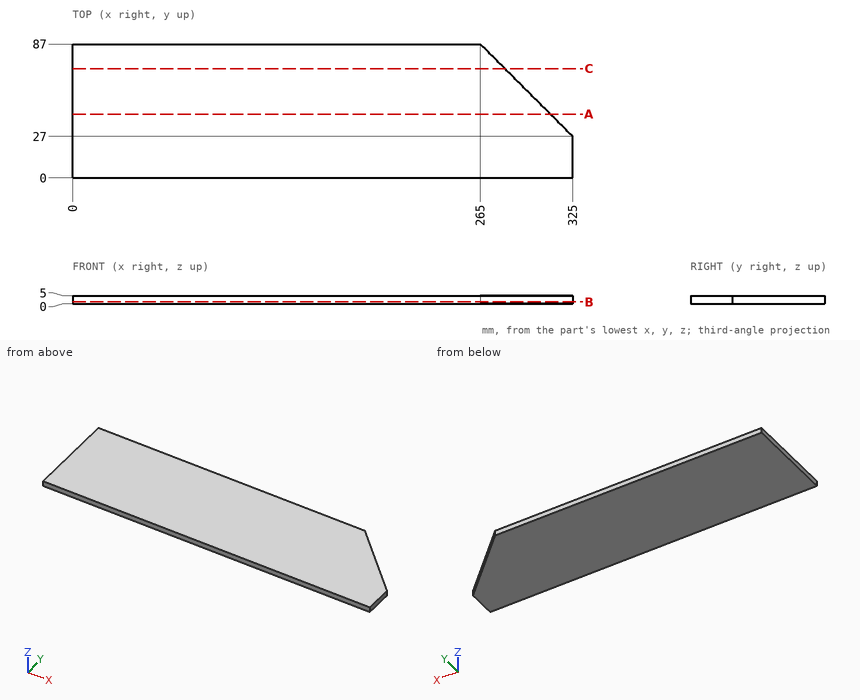
The drawing under review shows one solid part. Ordinate dimensions are in mm from its lowest x, y, z. Round coordinates to 2 decimals unless told otherwise and drop trailing zeros. Write each loop counter-clockwise with the first axis right and the second up, starting at its lowest first coordinate (ties: lowest second). Pieces come first, ordered by that corner, then holes.
(1) We need section A-A on y = 41.5. Give the boundary of the cut face in (x, z), and give its area (3 significant figures).
(2) Wall thickness on L1, parallel to X at y = 32.5, z = 2.4; L2, parallel to X at y = 61, z = 1.45; L3, parallel to Y at x = 301.5, z = 1.55: over which ranges is each line inside the solid? List them lowest first.
(3) We need section C-C on y = 71. Give the boundary of the cut face in (x, z), and give its area (4 significant figures).
(4) We need section B-B on z = 1.1. Give the boundary of the cut face in (x, y), and give its area (3 significant figures).
Findings below:
1. outline: (0, 0) - (310.5, 0) - (310.5, 5) - (0, 5) - close
1. area: 1,550 mm2
2. L1: x = 0 to 319.5
2. L2: x = 0 to 291
2. L3: y = 0 to 50.5
3. outline: (0, 0) - (281, 0) - (281, 5) - (0, 5) - close
3. area: 1,405 mm2
4. outline: (0, 0) - (325, 0) - (325, 27) - (265, 87) - (0, 87) - close
4. area: 26,500 mm2
